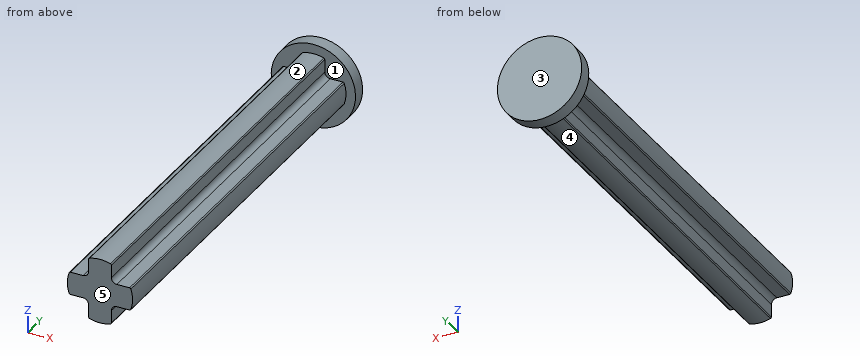
from build123d import *

# Parameters (mm, degrees)
SKETCH2_R           = 3.1
BOSS_EXTRUDE1_DEPTH = 31
SKETCH3_R           = 3.1
CUT_EXTRUDE1_DEPTH  = 30


with BuildPart() as part:
    # Sketch2 → Boss-Extrude1 (new body)
    with BuildSketch(Plane(origin=(0, 0, 0), x_dir=(1, 0, 0), z_dir=(0, 1, 0))):
        with Locations(Location((0, 0, 0), (0, 0, 270))):
            Circle(SKETCH2_R)
    extrude(amount=BOSS_EXTRUDE1_DEPTH)

    # Sketch3 → Cut-Extrude1 (cut)
    with BuildSketch(Plane(origin=(0, 0, 0), x_dir=(1, 0, 0), z_dir=(0, 1, 0))):
        with Locations(Location((0, 0, 0), (0, 0, 270))):
            Circle(SKETCH3_R)
        with BuildLine():
            Line((-0.84, -1.24), (-0.84, -2.177705214))
            ThreePointArc((-0.84, -2.177705214), (-0.821293884, -2.235940121), (-0.772173913, -2.27238805))
            ThreePointArc((-0.772173913, -2.27238805), (0, -2.4), (0.772173913, -2.27238805))
            ThreePointArc((0.772173913, -2.27238805), (0.821293884, -2.235940121), (0.84, -2.177705214))
            Line((0.84, -2.177705214), (0.84, -1.24))
            ThreePointArc((0.84, -1.24), (0.957157288, -0.957157288), (1.24, -0.84))
            Line((1.24, -0.84), (2.177705214, -0.84))
            ThreePointArc((2.177705214, -0.84), (2.235940121, -0.821293884), (2.27238805, -0.772173913))
            ThreePointArc((2.27238805, -0.772173913), (2.4, 0), (2.27238805, 0.772173913))
            ThreePointArc((2.27238805, 0.772173913), (2.235940121, 0.821293884), (2.177705214, 0.84))
            Line((2.177705214, 0.84), (1.24, 0.84))
            ThreePointArc((1.24, 0.84), (0.957157288, 0.957157288), (0.84, 1.24))
            Line((0.84, 1.24), (0.84, 2.177705214))
            ThreePointArc((0.84, 2.177705214), (0.821293884, 2.235940121), (0.772173913, 2.27238805))
            ThreePointArc((0.772173913, 2.27238805), (0, 2.4), (-0.772173913, 2.27238805))
            ThreePointArc((-0.772173913, 2.27238805), (-0.821293884, 2.235940121), (-0.84, 2.177705214))
            Line((-0.84, 2.177705214), (-0.84, 1.24))
            ThreePointArc((-0.84, 1.24), (-0.957157288, 0.957157288), (-1.24, 0.84))
            Line((-1.24, 0.84), (-2.177705214, 0.84))
            ThreePointArc((-2.177705214, 0.84), (-2.235940121, 0.821293884), (-2.27238805, 0.772173913))
            ThreePointArc((-2.27238805, 0.772173913), (-2.4, 0), (-2.27238805, -0.772173913))
            ThreePointArc((-2.27238805, -0.772173913), (-2.235940121, -0.821293884), (-2.177705214, -0.84))
            Line((-2.177705214, -0.84), (-1.24, -0.84))
            ThreePointArc((-1.24, -0.84), (-0.957157288, -0.957157288), (-0.84, -1.24))
        make_face(mode=Mode.SUBTRACT)
    extrude(amount=CUT_EXTRUDE1_DEPTH, mode=Mode.SUBTRACT)


solid = part.part
Build history of the part. All positions in model axes, mm. Face numbers are marked on the shaded views. A direction names the side the tool comes from. Coordinates: 2 decimals unless noted, no trailing zeros. Write each loop counter-clockwise with the first axis right and the second up, starting at its lowest first coordinate (ties: lowest second). Pieces come first, ordered by that corner, then holes.
(1) Drill centre lines: line 1 (Z direction, x = 2, y = 18.5); line 2 (Y direction, x = -2, z = 2.25). Where is each one in solid material? Low to high.
(2) Cut at B-B on x = 0. List the corners of the cut face in (y, z), and give its area (3 significant figures).
(3) Cut at A-A on z = 0. List the corners of the cut face in (x, y), and give its area (3 significant figures).
(4) Cut at C-C on y = 10. List the corners of the cut face in (x, z).
(5) 3-axis set-ups, long thin cutter, end or side, ignore diameter. For the marked faces 1, 2, 3, 4 and 5: which of +Z, -Z, +X, -X, +Y, -Y reach the whole face in a straight line?
(6) Pin check, flat tips, straight feed: pin 1 Ø0.5 at (x, y) = (-1.5, 19.5) entering from -Z; pin 2 Ø0.5 at (y, z) = (20, -2) entering from -X; pin 3 Ø0.5 at (x, y) = (-2, 16) entering from +Z. Stop position of each tip, or through.
Working result:
1. line 1: z = -0.84 to 0.84
1. line 2: y = 30 to 31
2. outline: (0, -2.4) - (30, -2.4) - (30, -3.1) - (31, -3.1) - (31, 3.1) - (30, 3.1) - (30, 2.4) - (0, 2.4) - close
2. area: 150 mm2
3. outline: (-3.1, 30) - (-2.4, 30) - (-2.4, 0) - (2.4, 0) - (2.4, 30) - (3.1, 30) - (3.1, 31) - (-3.1, 31) - close
3. area: 150 mm2
4. outline: (-2.27, -0.77) arc R0.1 ccw to (-2.18, -0.84) - (-1.24, -0.84) arc R0.4 cw to (-0.84, -1.24) - (-0.84, -2.18) arc R0.1 ccw to (-0.77, -2.27) arc R2.4 ccw to (0.77, -2.27) arc R0.1 ccw to (0.84, -2.18) - (0.84, -1.24) arc R0.4 cw to (1.24, -0.84) - (2.18, -0.84) arc R0.1 ccw to (2.27, -0.77) arc R2.4 ccw to (2.27, 0.77) arc R0.1 ccw to (2.18, 0.84) - (1.24, 0.84) arc R0.4 cw to (0.84, 1.24) - (0.84, 2.18) arc R0.1 ccw to (0.77, 2.27) arc R2.4 ccw to (-0.77, 2.27) arc R0.1 ccw to (-0.84, 2.18) - (-0.84, 1.24) arc R0.4 cw to (-1.24, 0.84) - (-2.18, 0.84) arc R0.1 ccw to (-2.27, 0.77) arc R2.4 ccw to start
5. face 1: -Y
5. face 2: +Z, -Y
5. face 3: +Z, -Z, +X, -X, +Y
5. face 4: -Z, -Y
5. face 5: +Z, -Z, +X, -X, -Y
6. pin 1: stops at z = -0.84
6. pin 2: stops at x = -0.84
6. pin 3: stops at z = 0.84
